from build123d import *

# Parameters (mm, degrees)
F0_R     = 38.110254
F1_DEPTH = 50.8
F2_R     = 36.885963
F2_R_2   = 13.436762
F3_DEPTH = 15.24
F5_D     = 24.13


with BuildPart() as f1:
    # F0 (on Top) → F1 (new body)
    with BuildSketch(Plane.XY):
        Circle(F0_R)
    extrude(amount=F1_DEPTH)

    # F2 (on Top) → F3 (cut)
    with BuildSketch(Plane.XY):
        Circle(F2_R)
        Circle(F2_R_2, mode=Mode.SUBTRACT)
    extrude(amount=F3_DEPTH, mode=Mode.SUBTRACT)

    # F5 (through all)
    with Locations(Plane(origin=(0, 0, 0), x_dir=(1, 0, 0), z_dir=(0, 0, -1))):
        with Locations((0, 0)):
            Hole(F5_D / 2)


solid = f1.part
Read the model definition and answer for the solid it produces. Units are mm, in the model's axes. A direction names the side the tool comes from. Give positions to 0.01 mm unless a question says otherwise; leave off trailing zeros. Write each loop counter-clockwise with the first axis right and the second up, starting at its lowest first coordinate (ties: lowest second). Pieces come first, ordered by that corner, then holes. Notation, with made-up numbers: (61.5, -39) -> (100.5, -39) arc R15 ccw to (100.5, -16) -> close; hole circle Ø8 at (-20, 49.25). An arc over 180 degrees is marked (long way). Answer as a JSON object with one key per item and string values. Group by question number.
1) Find section C-C (z = 8). Write down the section's boundary in (x, y) (1 decimal), and give its area (3 significant figures).
2) A tool of negligible diameter and unlimited length cuts with its end or side. For faces 4 (the flat face through (-9, 9, 50.8)), 5 (the flat face through (16, 1, 15.24)), from which of +Z, -Z, +X, -X, +Y, -Y can it reach the whole face along a straight path? Write none if from no direction.
3) Find section D-D (z = 27.5). Write down the section's boundary in (x, y) (1 decimal), and give its area (3 significant figures).
4) The mould has two halves that part along X. Classify faces 1 (the cylindrical face through (-4.961, 37.786, 25.044)), 2 (the cylindrical face through (-11.51, -3.62, 25.76)), 3 (the flat face through (-19.94, 31.23, 0)): +X half, -X half, draft (parallel to the pull), parting line (faces both ways), or undercut.
5) Find section A-A (x = 0). Write down the section's boundary in (y, z) (3 decimals).
6) Consider L1, parallel to Y at x = 0, z = 6 (3 decimals); L2, parallel to X at y = 4.5, z = 3; L3, parallel to Z at x = 12, y = 19.5. Determine where each line is inside the solid, lowest interval first. Write a range as from..to.
7) Each of these flat-tipped pins is pushed along its axis until it touches: P1, Ø5, axis at x = 5, y = -6, coming from the -Z side; P2, Ø12, axis at x = -17.5, z = 43, coming from the +Y side; P3, Ø8, axis at y = 8, z = 13, coming from the -X side; P4, Ø12, axis at x = -9.5, z = 6, coming from the -Y side. Where does it stop, or does it pass through?
Values follow:
{
 "1": {"outline": "circle Ø76.2 at (0, 0); circle Ø26.9 at (0, 0); hole circle Ø73.8 at (0, 0); hole circle Ø24.1 at (0, 0)", "area": "398 mm2"},
 "2": {"face 4": "+Z, +X, -X, +Y, -Y", "face 5": "-Z"},
 "3": {"outline": "circle Ø76.2 at (0, 0); hole circle Ø24.1 at (0, 0)", "area": "4,110 mm2"},
 "4": {"face 1": "parting line", "face 2": "undercut", "face 3": "draft"},
 "5": {"outline": "(-38.11, 0) -> (-36.886, 0) -> (-36.886, 15.24) -> (-13.437, 15.24) -> (-13.437, 0) -> (-12.065, 0) -> (-12.065, 50.8) -> (-38.11, 50.8) -> close; (12.065, 0) -> (13.437, 0) -> (13.437, 15.24) -> (36.886, 15.24) -> (36.886, 0) -> (38.11, 0) -> (38.11, 50.8) -> (12.065, 50.8) -> close"},
 "6": {"L1": "y = -38.11..-36.886, -13.437..-12.065, 12.065..13.437, 36.886..38.11", "L2": "x = -37.84..-36.61, -12.66..-11.19, 11.19..12.66, 36.61..37.84", "L3": "z = 15.24..50.8"},
 "7": {"P1": "passes through", "P2": "stops at y = 36.33", "P3": "stops at x = -37.9", "P4": "stops at y = -37.95"}
}
